For this review, take the finished solid that the model builds, in its own axes (mm). Face numbers are marked on the shaded views. A direction names the side the tool comes from. Coordinates: 2 decimals unless noted, no trailing zeros. Loops run counter-clockwise (first coordinate to the right, second up) from the corner with the lowest first, then second, coordinate; pieces in that order, holes last. Notation, with made-up numbers: (68, 17.25) - (105, 17.25) arc R16 cw to (105, 24.25) - close; hole circle Ø4 at (-23, -38). An arc over 180 degrees is marked (long way). Answer as a JSON object with one key per item and string values. Group by question number.
Item 1: We need section A-A (x = 3). Give the boundary of the cut face in (y, z).
Item 2: We need section B-B (y = 14.5). Give the boundary of the cut face in (x, z), then the cut area to 3 significant figures.
Item 3: Clearance check with flat-ended pins moving along their axes: pin 1 (12 mm diameter, centred on x = 26.5, y = 3.5, fed in from +Z); pin 2 (9.5 mm diameter, centred on x = 15.5, z = 26, fed in from -Y); pin 3 (10 mm diameter, centred on x = 17, y = 18, fed in from +Z). State where each tip first meets the part, or that it passes through.
Item 4: To check wall thickness, follow line 1 (X direction, y = 19.25, z = 28.5); line 2 (Z direction, x = 30, y = 5.25); line 3 (Y direction, x = 15, z = 20). State the ranges of each line that lie inside material, in increasing order.
Item 5: We need section D-D (x = 14). Give the boundary of the cut face in (y, z).
Item 6: We need section C-C (z = 22.5). Give the boundary of the cut face in (x, y), then the cut area to 3 significant figures.
Item 7: Tool access review of the marked faces 1, 2 and 3: name each direction out of +Z, -Z, +X, -X, +Y, -Y from which nothing blocks a thin tool from reaching the whole face with its end or side.
from build123d import *

# Parameters (mm, degrees)
F1_DEPTH = 31.75
F2_W     = 12.7
F2_H     = 6.35
F3_DEPTH = 25.4
F4_DEPTH = 25.4


with BuildPart() as f1:
    # F0 (on Right) → F1 (new body)
    with BuildSketch(Plane.YZ):
        Polygon((0, 12.7), (0, 0), (25.4, 0), (25.4, 31.75), (12.7, 31.75), (12.7, 12.7), align=None)
    extrude(amount=F1_DEPTH)

    # F2 (on Front) → F3 (cut)
    with BuildSketch(Plane.XZ):
        with Locations((15.830855, 29.134337)):
            Rectangle(F2_W, F2_H)
    extrude(amount=-F3_DEPTH, mode=Mode.SUBTRACT)

    # F2 (on Front) → F4 (cut)
    with BuildSketch(Plane.XZ):
        with Locations((15.830855, 29.134337)):
            Rectangle(F2_W, F2_H)
    extrude(amount=-F4_DEPTH, mode=Mode.SUBTRACT)


solid = f1.part
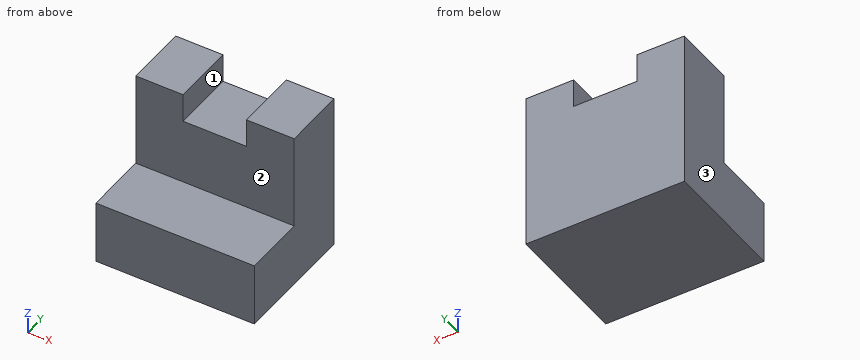
Check sheet entries:
{
 "1": {"outline": "(0, 0) - (25.4, 0) - (25.4, 31.75) - (12.7, 31.75) - (12.7, 12.7) - (0, 12.7) - close"},
 "2": {"outline": "(0, 0) - (31.75, 0) - (31.75, 31.75) - (22.18, 31.75) - (22.18, 25.96) - (9.48, 25.96) - (9.48, 31.75) - (0, 31.75) - close", "area": "935 mm2"},
 "3": {"pin 1": "stops at z = 12.7", "pin 2": "stops at y = 12.7", "pin 3": "stops at z = 25.96"},
 "4": {"line 1": "x = 0 to 9.48, 22.18 to 31.75", "line 2": "z = 0 to 12.7", "line 3": "y = 12.7 to 25.4"},
 "5": {"outline": "(0, 0) - (25.4, 0) - (25.4, 25.96) - (12.7, 25.96) - (12.7, 12.7) - (0, 12.7) - close"},
 "6": {"outline": "(0, 12.7) - (31.75, 12.7) - (31.75, 25.4) - (0, 25.4) - close", "area": "403 mm2"},
 "7": {"face 1": "+Z, +Y, -Y", "face 2": "+Z, +X, -X, -Y", "face 3": "+Z, -Z, -X, +Y, -Y"}
}
